```python
from build123d import *

# Parameters (mm, degrees)
SKETCH_1_R          = 1.45
EXTRUDE_1_DEPTH     = 3
FILLET_1_R          = 2
SKETCH_2_R          = 1.6
CUT_EXTRUDE_1_DEPTH = 78.839578622


with BuildPart() as part:
    # 草图1 → 凸台-拉伸1 (new body)
    with BuildSketch(Plane(origin=(0, 0, 0), x_dir=(1, 0, 0), z_dir=(0, 1, 0))):
        Polygon((-55, 0), (0, 0), (0, -55), (-15, -55), (-15, -15), (-55, -15), align=None)
        with Locations(Location((-7.5, -7.5, 0), (0, 0, 270))):
            Circle(SKETCH_1_R, mode=Mode.SUBTRACT)
        with Locations(Location((-7.5, -30, 0), (0, 0, 270))):
            Circle(SKETCH_1_R, mode=Mode.SUBTRACT)
        with Locations(Location((-7.5, -50, 0), (0, 0, 270))):
            Circle(SKETCH_1_R, mode=Mode.SUBTRACT)
        with Locations(Location((-30, -7.5, 0), (0, 0, 270))):
            Circle(SKETCH_1_R, mode=Mode.SUBTRACT)
        with Locations(Location((-50, -7.5, 0), (0, 0, 270))):
            Circle(SKETCH_1_R, mode=Mode.SUBTRACT)
    extrude(amount=EXTRUDE_1_DEPTH)

    # 圆角1
    fillet_1_edges = [part.edges().sort_by_distance(p)[0] for p in [
        (-55, 1.5, 0),
        (0, 1.5, 0),
        (0, 1.5, 55),
        (-15, 1.5, 55),
        (-55, 1.5, 15),
    ]]
    fillet(fillet_1_edges, radius=FILLET_1_R)

    # 草图2 → 切除-拉伸1 (cut, through all)
    with BuildSketch(Plane(origin=(0, 3, 0), x_dir=(1, 0, 0), z_dir=(0, 1, 0))):
        with Locations((-15, -15)):
            Circle(SKETCH_2_R)
    extrude(amount=-CUT_EXTRUDE_1_DEPTH, mode=Mode.SUBTRACT)


solid = part.part
```
Read the model definition and answer for the solid it produces. Units are mm, in the model's axes. A direction names the side the tool comes from. Give positions to 0.01 mm unless a question says otherwise; leave off trailing zeros. Order: outer loops, then holes, each group sorted by start corner. A loop starts at its lowest first (then second) coordinate and runs counter-clockwise, first axis right, second up.
(1) For faces 1 (the flat face through (-35, 1, 15)), 2 (the flat face through (-21, 0, 9)), determine the directions among +Z, -Z, +X, -X, +Y, -Y from which every point of the face is accessible in a straight line to the end or side of a thin tool.
(2) Straight lines are drawn through the part: L1, parallel to X at y = 2.05, z = 7.5; L2, parallel to Z at x = -8.5, y = 1.8; L3, parallel to Z at x = -33, y = 0.5. For each, find the intervals that lie inside material, in ascending order.
(3) Find section C-C (x = -7.5). Give the vertices of the cut face in (y, z).
(4) Find section B-B (y = 0.5). Give the vertices of the cut face in (x, z).
(5) Given pin 1 (0.9 mm diameter, centred on y = 1, z = 44, fed in from -X); pin 2 (1 mm diameter, centred on x = -25.5, y = 1.5, fed in from +Z), each flat-ended and moving along its own axis, determine where each tip first touches the part or whether it passes through.
(6) For a pull along Z with two mould halves and no side action, classify faces 3 (the flat face through (-55, 1, 8)), 4 (the cylindrical face through (-50.88, 1.48, 6.35)), 5 (the cylindrical face through (-14.4, 1.52, 54.43)) as released by +Z, released by -Z, zero draft, split by the parting line, or undercut.
(7) Find section D-D (x = -27.5). Give the vertices of the cut face in (y, z), plus the area to 3 significant figures.
(8) Find section A-A (z = 30). Give the vertices of the cut face in (x, y), plus the area to 3 significant figures.
Result sheet:
1. face 1: +Z, -X, +Y, -Y
1. face 2: +Z, -Z, +X, -X, -Y
2. L1: x = -55 to -51.45, -48.55 to -31.45, -28.55 to -8.95, -6.05 to 0
2. L2: z = 0 to 6.45, 8.55 to 28.95, 31.05 to 48.95, 51.05 to 55
2. L3: z = 0 to 15
3. outline: (0, 0) - (3, 0) - (3, 6.05) - (0, 6.05) - close; (0, 8.95) - (3, 8.95) - (3, 28.55) - (0, 28.55) - close; (0, 31.45) - (3, 31.45) - (3, 48.55) - (0, 48.55) - close; (0, 51.45) - (3, 51.45) - (3, 55) - (0, 55) - close
4. outline: (-55, 2) arc R2 ccw to (-53, 0) - (-2, 0) arc R2 ccw to (0, 2) - (0, 53) arc R2 ccw to (-2, 55) - (-13, 55) arc R2 ccw to (-15, 53) - (-15, 16.6) arc R1.6 cw (long way) to (-16.6, 15) - (-53, 15) arc R2 ccw to (-55, 13) - close; hole circle Ø2.9 at (-50, 7.5); hole circle Ø2.9 at (-30, 7.5); hole circle Ø2.9 at (-7.5, 7.5); hole circle Ø2.9 at (-7.5, 30); hole circle Ø2.9 at (-7.5, 50)
5. pin 1: stops at x = -15
5. pin 2: stops at z = 15
6. face 3: zero draft
6. face 4: undercut
6. face 5: released by +Z
7. outline: (0, 0) - (3, 0) - (3, 15) - (0, 15) - close
7. area: 45.0 mm2
8. outline: (-15, 0) - (-8.95, 0) - (-8.95, 3) - (-15, 3) - close; (-6.05, 0) - (0, 0) - (0, 3) - (-6.05, 3) - close
8. area: 36.3 mm2
